Work out the finished part from the listing and answer in its coordinate system (mm). Coordinates: 2 decimals unless noted, no trailing zeros. Write each loop counter-clockwise with the first axis right and the second up, starting at its lowest first coordinate (ties: lowest second). Pieces come first, ordered by that corner, then holes. Notation, with made-up numbers: (73, 64.25) - (115, 64.25) arc R26 ccw to (115, 85.25) - close; hole circle Ø7 at (-17, 2.5). An arc over 180 degrees is marked (long way). Use one line per item in the form item = value. Start each with the question number.
Item 1: A cutting plane is placed at B-B (z = 11.25). Give the number of separate pieces and of enclosed holes in the cut face, then the cut area to 3 significant figures.
Item 2: Consider probe 1 along X at (y, z) = (-0.45, 14); probe 2 along X at (y, z) = (-0.65, -48.5); probe 3 along Z at (x, y) = (-9, -0.85). Determine where each line is inside the solid, lowest interval first.
Item 3: Determine the mould class of faces 1 (the flat face through (-1, -2, -12)), 2 (the cylindrical face through (27.44, -0.99, -34.66)), 3 (the cylindrical face through (-17.25, -0.99, -11.18)) for opening direction X: released by +X, released by -X, zero draft, split by the parting line, or undercut.
Item 4: Given pin 1 (1.8 mm diameter, centred on x = -18.75, z = -26.25, fed in from +Y), flat-ended and moving along its own axis, determine where the tip first touches the part or whether it passes through.
Item 5: A cutting plane is placed at A-A (z = -50). Write down the section's boundary in (x, y), then the cut area to 3 significant figures.
from build123d import *

# Parameters (mm, degrees)
F0_W      = 100
F0_H      = 120
F0_R      = 2
F1_DEPTH  = 2
F2_W      = 22
F2_H      = 60
F3_DEPTH  = 2.001
F4_R      = 1.5
F5_R      = 1.5
F6_DEPTH  = 2.001
F7_R      = 1.5
F8_DEPTH  = 2.001
F9_R      = 2.25
F10_DEPTH = 2.001
F12_DEPTH = 2.001


with BuildPart() as f1:
    # F0 (on Front) → F1 (new body)
    with BuildSketch(Plane.XZ):
        Rectangle(F0_W, F0_H)
        with Locations((-40, -50)):
            Circle(F0_R, mode=Mode.SUBTRACT)
        with Locations((40, -50)):
            Circle(F0_R, mode=Mode.SUBTRACT)
        with Locations((-40, 50)):
            Circle(F0_R, mode=Mode.SUBTRACT)
        with Locations((40, 50)):
            Circle(F0_R, mode=Mode.SUBTRACT)
    extrude(amount=F1_DEPTH)

    # F2 (on face) → F3 (cut, through all)
    with BuildSketch(Plane.XZ.offset(2)):
        with Locations((0, 30)):
            Rectangle(F2_W, F2_H)
    extrude(amount=-F3_DEPTH, mode=Mode.SUBTRACT)

    # F4
    f4_edges = [f1.edges().sort_by_distance(p)[0] for p in [
        (-11, -1, 0),
        (11, -1, 0),
        (-11, -1, 60),
        (11, -1, 60),
    ]]
    fillet(f4_edges, radius=F4_R)

    # F5 (on face) → F6 (cut, through all)
    with BuildSketch(Plane(origin=(0, 0, 0), x_dir=(-1, 0, 0), z_dir=(0, 1, 0))):
        with Locations((33.75, 33.75)):
            Circle(F5_R)
        with Locations((33.75, 26.25)):
            Circle(F5_R)
        with Locations((33.75, 18.75)):
            Circle(F5_R)
        with Locations((33.75, 11.25)):
            Circle(F5_R)
        with Locations((33.75, 3.75)):
            Circle(F5_R)
        with Locations((33.75, -3.75)):
            Circle(F5_R)
        with Locations((33.75, -11.25)):
            Circle(F5_R)
        with Locations((33.75, -18.75)):
            Circle(F5_R)
        with Locations((33.75, -26.25)):
            Circle(F5_R)
        with Locations((33.75, -33.75)):
            Circle(F5_R)
        with Locations((26.25, 33.75)):
            Circle(F5_R)
        with Locations((26.25, 26.25)):
            Circle(F5_R)
        with Locations((26.25, 18.75)):
            Circle(F5_R)
        with Locations((26.25, 11.25)):
            Circle(F5_R)
        with Locations((26.25, 3.75)):
            Circle(F5_R)
        with Locations((26.25, -3.75)):
            Circle(F5_R)
        with Locations((26.25, -11.25)):
            Circle(F5_R)
        with Locations((26.25, -18.75)):
            Circle(F5_R)
        with Locations((26.25, -26.25)):
            Circle(F5_R)
        with Locations((26.25, -33.75)):
            Circle(F5_R)
        with Locations((18.75, 26.25)):
            Circle(F5_R)
        with Locations((18.75, 18.75)):
            Circle(F5_R)
        with Locations((18.75, 11.25)):
            Circle(F5_R)
        with Locations((18.75, 3.75)):
            Circle(F5_R)
        with Locations((18.75, -3.75)):
            Circle(F5_R)
        with Locations((18.75, -11.25)):
            Circle(F5_R)
        with Locations((18.75, -18.75)):
            Circle(F5_R)
        with Locations((18.75, -26.25)):
            Circle(F5_R)
        with Locations((-26.25, 18.75)):
            Circle(F5_R)
        with Locations((-26.25, 3.75)):
            Circle(F5_R)
        with Locations((-18.75, -18.75)):
            Circle(F5_R)
        with Locations((-33.75, -26.25)):
            Circle(F5_R)
        with Locations((-33.75, 18.75)):
            Circle(F5_R)
        with Locations((-26.25, 26.25)):
            Circle(F5_R)
        with Locations((-26.25, 33.75)):
            Circle(F5_R)
        with Locations((-33.75, 33.75)):
            Circle(F5_R)
        with Locations((-18.75, 3.75)):
            Circle(F5_R)
        with Locations((-33.75, 3.75)):
            Circle(F5_R)
        with Locations((-26.25, -3.75)):
            Circle(F5_R)
        with Locations((-33.75, -33.75)):
            Circle(F5_R)
        with Locations((-26.25, -26.25)):
            Circle(F5_R)
        with Locations((-33.75, -11.25)):
            Circle(F5_R)
        with Locations((-26.25, -11.25)):
            Circle(F5_R)
        with Locations((-33.75, -3.75)):
            Circle(F5_R)
        with Locations((-33.75, 26.25)):
            Circle(F5_R)
        with Locations((-18.75, 11.25)):
            Circle(F5_R)
        with Locations((-18.75, 18.75)):
            Circle(F5_R)
        with Locations((-18.75, -11.25)):
            Circle(F5_R)
        with Locations((-18.75, 26.25)):
            Circle(F5_R)
        with Locations((-26.25, -18.75)):
            Circle(F5_R)
        with Locations((-33.75, -18.75)):
            Circle(F5_R)
        with Locations((-26.25, 11.25)):
            Circle(F5_R)
        with Locations((-18.75, -26.25)):
            Circle(F5_R)
        with Locations((-33.75, 11.25)):
            Circle(F5_R)
        with Locations((-18.75, -3.75)):
            Circle(F5_R)
        with Locations((-26.25, -33.75)):
            Circle(F5_R)
    extrude(amount=-F6_DEPTH, mode=Mode.SUBTRACT)

    # F7 (on face) → F8 (cut, through all)
    with BuildSketch(Plane.XZ.offset(2)):
        with Locations((-41.25, 33.75)):
            Circle(F7_R)
        with Locations((-41.25, 26.25)):
            Circle(F7_R)
        with Locations((-41.25, 18.75)):
            Circle(F7_R)
        with Locations((-41.25, 11.25)):
            Circle(F7_R)
        with Locations((-41.25, 3.75)):
            Circle(F7_R)
        with Locations((-41.25, -3.75)):
            Circle(F7_R)
        with Locations((-41.25, -11.25)):
            Circle(F7_R)
        with Locations((-41.25, -18.75)):
            Circle(F7_R)
        with Locations((-41.25, -26.25)):
            Circle(F7_R)
        with Locations((-41.25, -33.75)):
            Circle(F7_R)
        with Locations((41.25, -26.25)):
            Circle(F7_R)
        with Locations((41.25, -18.75)):
            Circle(F7_R)
        with Locations((41.25, -11.25)):
            Circle(F7_R)
        with Locations((41.25, 18.75)):
            Circle(F7_R)
        with Locations((41.25, -3.75)):
            Circle(F7_R)
        with Locations((41.25, 26.25)):
            Circle(F7_R)
        with Locations((41.25, 33.75)):
            Circle(F7_R)
        with Locations((41.25, 3.75)):
            Circle(F7_R)
        with Locations((41.25, 11.25)):
            Circle(F7_R)
        with Locations((41.25, -33.75)):
            Circle(F7_R)
    extrude(amount=-F8_DEPTH, mode=Mode.SUBTRACT)

    # F9 (on face) → F10 (cut, through all)
    with BuildSketch(Plane(origin=(0, 0, 0), x_dir=(-1, 0, 0), z_dir=(0, 1, 0))):
        with Locations((-26.25, 33.75)):
            Circle(F9_R)
    extrude(amount=-F10_DEPTH, mode=Mode.SUBTRACT)

    # F11 (on face) → F12 (cut, through all)
    with BuildSketch(Plane(origin=(0, 0, 0), x_dir=(-1, 0, 0), z_dir=(0, 1, 0))):
        with BuildLine():
            ThreePointArc((-18.85, 50), (-16.75, 47.9), (-14.65, 50))
            ThreePointArc((-14.65, 50), (-16.75, 52.1), (-18.85, 50))
        make_face()
    extrude(amount=-F12_DEPTH, mode=Mode.SUBTRACT)


solid = f1.part
Answer:
q1.separate_pieces = 10
q1.enclosed_holes = 0
q1.area = 108 mm²
q2.probe_1 = -50 to -11, 11 to 50
q2.probe_2 = -50 to -41.32, -38.68 to 38.68, 41.32 to 50
q2.probe_3 = -60 to 0
q3.face_1 = zero draft
q3.face_2 = undercut
q3.face_3 = undercut
q4.pin_1 = through
q5.outline = (-50, -2) - (-42, -2) - (-42, 0) - (-50, 0) - close; (-38, -2) - (38, -2) - (38, 0) - (-38, 0) - close; (42, -2) - (50, -2) - (50, 0) - (42, 0) - close
q5.area = 184 mm²
